Build history of the part. All positions in model axes, mm. A direction names the side the tool comes from. Round coordinates to 2 decimals unless told otherwise and drop trailing zeros. Loops run counter-clockwise (first coordinate to the right, second up) from the corner with the lowest first, then second, coordinate; pieces in that order, holes last. Notation, with made-up numbers: (42.5, 34.25) -> (52.5, 34.25) arc R20 ccw to (52.5, 53.25) -> close; hole circle Ø4 at (80.25, -38.5). An arc over 180 degrees is marked (long way). Put each result on its own line as item: value. Start each with the question number.
Autodesk Inventor part; units mm, degrees
ref_plane "YZ Plane" through (0, 0, 0) normal (1, 0, 0) x (0, 1, 0)
ref_plane "XZ Plane" through (0, 0, 0) normal (0, 1, 0) x (-1, 0, 0)
ref_plane "XY Plane" through (0, 0, 0) normal (0, 0, 1) x (1, 0, 0)
sketch "Skizze1" plane through (0, 0, 0) normal (0, 1, 0) x (-1, 0, 0)
  line L0 (-50, 40) -> (50, 40)
  line L1 (50, 40) -> (50, -40)
  line L2 (50, -40) -> (-50, -40)
  line L3 (-50, -40) -> (-50, 40)
  line L4 (-50, 40) -> (50, -40) construction
  line L5 (50, 40) -> (-50, -40) construction
  point P0 (0, 0)
  dimension "d0" = 100
  dimension "d1" = 80
extrude "Extrusion1" add sketch "Skizze1" along normal blind 5
sketch "Skizze2" plane through (0, 5, 0) normal (0, 1, 0) x (1, 0, 0)
  line L0 (-50, -40) -> (50, -40)
  line L1 (50, -40) -> (50, 40)
  line L2 (50, 40) -> (-50, 40)
  line L3 (-50, 40) -> (-50, -40)
  line L4 (-45, -35) -> (45, -35)
  line L5 (45, -35) -> (45, 35)
  line L6 (45, 35) -> (-45, 35)
  line L7 (-45, 35) -> (-45, -35)
  line L8 (-45, -35) -> (45, 35) construction
  line L9 (45, -35) -> (-45, 35) construction
  point P0 (0, 0)
  dimension "d4" = 90
  dimension "d5" = 70
extrude "Extrusion2" add sketch "Skizze2" along normal blind 15
sketch "Skizze3" plane through (0, 20, 0) normal (0, 1, 0) x (1, 0, 0)
  line L0 (47.75, -37.75) -> (-47.75, -37.75)
  line L1 (-47.75, -37.75) -> (-47.75, 37.75)
  line L2 (-47.75, 37.75) -> (47.75, 37.75)
  line L3 (47.75, 37.75) -> (47.75, -37.75)
  line L4 (47.75, -37.75) -> (-47.75, 37.75) construction
  line L5 (-47.75, -37.75) -> (47.75, 37.75) construction
  line L6 (-45, 35) -> (-45, -35)
  line L7 (-45, -35) -> (45, -35)
  line L8 (45, -35) -> (45, 35)
  line L9 (45, 35) -> (-45, 35)
  point P0 (0, 0)
  dimension "d8" = 95.5
  dimension "d9" = 75.5
extrude "Extrusion3" cut sketch "Skizze3" against normal blind 6
properties part number "bottom"
Item 1: Wall check: line 1 (Z direction, x = 30, y = 12.5); line 2 (X direction, y = 11.5, z = -24); line 3 (Z direction, x = 11, y = 18.5). Give the ranges that are in metal, low to high. Write a range as from..to.
Item 2: 3-axis set-ups, long thin cutter, end or side, ignore diameter. For faces 1 (the face through (1, 5, 0)), 2 (the face through (1, 10, 40)): which of +Z, -Z, +X, -X, +Y, -Y reach the whole face in a straight line?
Item 3: Drop a flat-ended pin along its axis: pin 1 (5 mm diameter, centred on x = 0.5, z = 6, fed in from +Y). Give the stop position or say it passes through.
Item 4: Cut at A-A on y = 16.75. Write the cut outline in (x, z).
Item 5: Cut at C-C on z = 30.5. Write the cut outline in (x, y), then the cut area to 3 significant figures.
Item 6: Cut at D-D on y = 7.5. Write the cut outline in (x, z), then the cut area to 3 significant figures.
Item 7: Cut at B-B on x = 26.5. Write the cut outline in (y, z).
Item 8: Pull direction Z, two halves, no side cores. Call faces 3 (the face through (-4, 14, 36)), 4 (the face through (-4, 20, 38)), 5 (the face through (-1, 10, -40)): +Z half, -Z half, draft (parallel to the pull), parting line (faces both ways), or undercut.
Ans:
1. line 1: z = -40..-35, 35..40
1. line 2: x = -50..-45, 45..50
1. line 3: z = -40..-37.75, 37.75..40
2. face 1: +Y
2. face 2: +Z, +X, -X, +Y, -Y
3. pin 1: stops at y = 5
4. outline: (-50, -40) -> (50, -40) -> (50, 40) -> (-50, 40) -> close; hole (-47.75, -37.75) -> (47.75, -37.75) -> (47.75, 37.75) -> (-47.75, 37.75) -> close
5. outline: (-50, 0) -> (50, 0) -> (50, 20) -> (47.75, 20) -> (47.75, 14) -> (45, 14) -> (45, 5) -> (-45, 5) -> (-45, 14) -> (-47.75, 14) -> (-47.75, 20) -> (-50, 20) -> close
5. area: 617 mm2
6. outline: (-50, -40) -> (50, -40) -> (50, 40) -> (-50, 40) -> close; hole (-45, -35) -> (45, -35) -> (45, 35) -> (-45, 35) -> close
6. area: 1,700 mm2
7. outline: (0, -40) -> (20, -40) -> (20, -37.75) -> (14, -37.75) -> (14, -35) -> (5, -35) -> (5, 35) -> (14, 35) -> (14, 37.75) -> (20, 37.75) -> (20, 40) -> (0, 40) -> close
8. face 3: undercut
8. face 4: draft
8. face 5: -Z half
